Autodesk Inventor part; units mm, degrees
ref_plane "YZ Plane" through (0, 0, 0) normal (1, 0, 0) x (0, 1, 0)
ref_plane "XZ Plane" through (0, 0, 0) normal (0, 1, 0) x (-1, 0, 0)
ref_plane "XY Plane" through (0, 0, 0) normal (0, 0, 1) x (1, 0, 0)
sketch "Sketch1" plane through (0, 0, 0) normal (0, 1, 0) x (-1, 0, 0)
  circle A0 centre (0, 0) radius 177
  dimension "d0" = 354
extrude "Extrusion1" add sketch "Sketch1" along normal blind 5
sketch "Sketch2" plane through (0, 5, 0) normal (0, 1, 0) x (1, 0, 0)
  line L0 (0, 0) -> (153.2865, -88.5) construction
  circle A0 centre (0, 0) radius 177 construction
  line L1 (-177, 0) -> (177, 0) construction
  circle A1 centre (142.288, -82.15) radius 1.7
  line L2 (142.288, -82.15) -> (134.0391, -77.3875) construction
  circle A2 centre (142.288, -72.625) radius 1.7
  circle A3 centre (134.0391, -67.8625) radius 1.7
  circle A4 centre (125.7902, -72.625) radius 1.7
  circle A5 centre (125.7902, -82.15) radius 1.7
  circle A6 centre (134.0391, -86.9125) radius 1.7
  circle A7 centre (142.288, 82.15) radius 1.7
  circle A8 centre (142.288, 72.625) radius 1.7
  circle A9 centre (134.0391, 67.8625) radius 1.7
  circle A10 centre (125.7902, 72.625) radius 1.7
  circle A11 centre (125.7902, 82.15) radius 1.7
  circle A12 centre (134.0391, 86.9125) radius 1.7
  line L3 (0, 177) -> (0, -177) construction
  circle A13 centre (0, 0) radius 177 construction
  circle A14 centre (-142.288, -82.15) radius 1.7
  circle A15 centre (-142.288, -72.625) radius 1.7
  circle A16 centre (-134.0391, -67.8625) radius 1.7
  circle A17 centre (-125.7902, -72.625) radius 1.7
  circle A18 centre (-125.7902, -82.15) radius 1.7
  circle A19 centre (-134.0391, -86.9125) radius 1.7
  circle A20 centre (-134.0391, 67.8625) radius 1.7
  circle A21 centre (-142.288, 72.625) radius 1.7
  circle A22 centre (-142.288, 82.15) radius 1.7
  circle A23 centre (-134.0391, 86.9125) radius 1.7
  circle A24 centre (-125.7902, 82.15) radius 1.7
  circle A25 centre (-125.7902, 72.625) radius 1.7
  dimension "d3" = 30
  dimension "d4" = 3.4
  dimension "d5" = 12.7
  dimension "d6" = 9.525
  dimension "d9" = 360
extrude "Standoffs" cut sketch "Sketch2" against normal through all
sketch "Sketch3" plane through (0, 5, 0) normal (0, 1, 0) x (1, 0, 0)
  circle A0 centre (-127, 50.8) radius 10.16
  circle A1 centre (127, 50.8) radius 10.16
  circle A2 centre (0, 0) radius 177 construction
  circle A3 centre (0, 0) radius 177 construction
  line L0 (0, 0) -> (0, 177) construction
  line L1 (0, 0) -> (177, 0) construction
  line L2 (0, 0) -> (-177, 0) construction
  dimension "d13" = 20.32
  dimension "d14" = 20.32
  dimension "d19" = 127
  dimension "d20" = 127
  dimension "d21" = 50.8
  dimension "d22" = 50.8
extrude "Wires" cut sketch "Sketch3" against normal through all
sketch "Sketch4" plane through (0, 5, 0) normal (0, 1, 0) x (1, 0, 0)
  circle A0 centre (0, -141.44) radius 2.667
  circle A1 centre (0, 0) radius 177 construction
  line L0 (0, 0) -> (0, -177) construction
  line L1 (0, -177) -> (48.7641, -177) construction
  circle A2 centre (100.0132, -100.0132) radius 2.667
  circle A3 centre (141.44, 0) radius 2.667
  circle A4 centre (100.0132, 100.0132) radius 2.667
  circle A5 centre (0, 141.44) radius 2.667
  circle A6 centre (-100.0132, 100.0132) radius 2.667
  circle A7 centre (-141.44, 0) radius 2.667
  circle A8 centre (-100.0132, -100.0132) radius 2.667
  dimension "d25" = 5.334
  dimension "d28" = 35.56
  dimension "d31" = 360
extrude "Zip Ties" cut sketch "Sketch4" against normal through all
equation "\"d0\" = robot_diameter"
equation "\"d1\" = hardboard_thickness"
equation "\"d4\" = m3_clearance"
equation "\"d14\" = d13"
equation "\"d22\" = d21"
equation "\"m3_heat_set_insert\" = 4"
equation "\"m3_clearance\" = 3.4"
equation "\"m3_heat_set_depth\" = 7"
equation "\"robot_diameter\" = 354"
equation "\"hardboard_thickness\" = 5"
properties part number "layer5_new"
Read the model definition and answer for the solid it produces. Units are mm, in the model's axes. Round coordinates to 2 decimals unless told otherwise and drop trailing zeros. Loops run counter-clockwise (first coordinate to the right, second up) from the corner with the lowest first, then second, coordinate; pieces in that order, holes last. Notation, with made-up numbers: (28.25, 76.25) - (69.25, 76.25) arc R15 cw to (69.25, 89.25) - close; hole circle Ø10 at (15, 14.5). An arc over 180 degrees is marked (long way). One line per question, with ' | ' between items. Start each with the question number.
Q1. For a pull along Z with two mould halves and no side action, classify faces 1 (the flat face through (2, 0, 2)), 2 (the cylindrical face through (38.37, 2.46, 172.79)), 3 (the cylindrical face through (125.677, 2.535, -60.874)) as +Z half, -Z half, draft (parallel to the pull), parting line (faces both ways), or undercut.
Q2. Section D-D on x = -50.5 is taken. Give the vertices of the cut face in (y, z).
Q3. Find the intervals of material crossed by L1, parallel to Z at x = 0.5, y = 2.55; L2, parallel to X at y = 3.15, z = 82.15; L3, parallel to Z at x = -2, y = 2.45, in increasing order.
Q4. Flat-ended cylindrical pins translate along their axes: pin 1 (1.5 mm diameter, centred on y = 4, z = 82, fed in from -X); pin 2 (2 mm diameter, centred on y = 4.5, z = 45, fed in from +X). Find the tip coordinate at first contact, or state that the pin passes through.
Q5. Section B-B on z = 154.5 is taken. Give the vertices of the cut face in (x, y), plus the area to 3 significant figures.
Q6. Section A-A on z = -50.8 is taken. Give the vertices of the cut face in (x, y).
Q7. Section C-C on y = 1.3 is taken. Count the separate pieces of the cut face and the enclosed holes in it, plus the area to 3 significant figures.
Established:
1) face 1: draft | face 2: parting line | face 3: undercut
2) outline: (0, -169.64) - (5, -169.64) - (5, 169.64) - (0, 169.64) - close
3) L1: -177 to -144.06, -138.82 to 138.82, 144.06 to 177 | L2: -156.78 to -143.99, -140.59 to -127.49, -124.09 to 124.09, 127.49 to 140.59, 143.99 to 156.78 | L3: -176.99 to -143.2, -139.68 to 139.68, 143.2 to 176.99
4) pin 1: x = -157.25 | pin 2: x = 171.44
5) outline: (-86.36, 0) - (86.36, 0) - (86.36, 5) - (-86.36, 5) - close | area: 864 mm²
6) outline: (-169.55, 0) - (-137.16, 0) - (-137.16, 5) - (-169.55, 5) - close; (-116.84, 0) - (116.84, 0) - (116.84, 5) - (-116.84, 5) - close; (137.16, 0) - (169.55, 0) - (169.55, 5) - (137.16, 5) - close
7) separate pieces: 1 | enclosed holes: 34 | area: 97,400 mm²
